For this review, use the dimensioned drawing (mm, ordinates from the lowest corner) and the shaded views. A direction names the side the tool comes from. Coordinates: 2 decimals unless noted, no trailing zeros. Write each loop counter-clockwise with the first axis right and the second up, starting at its lowest first coordinate (ties: lowest second). Pieces come first, ordered by that corner, then holes.
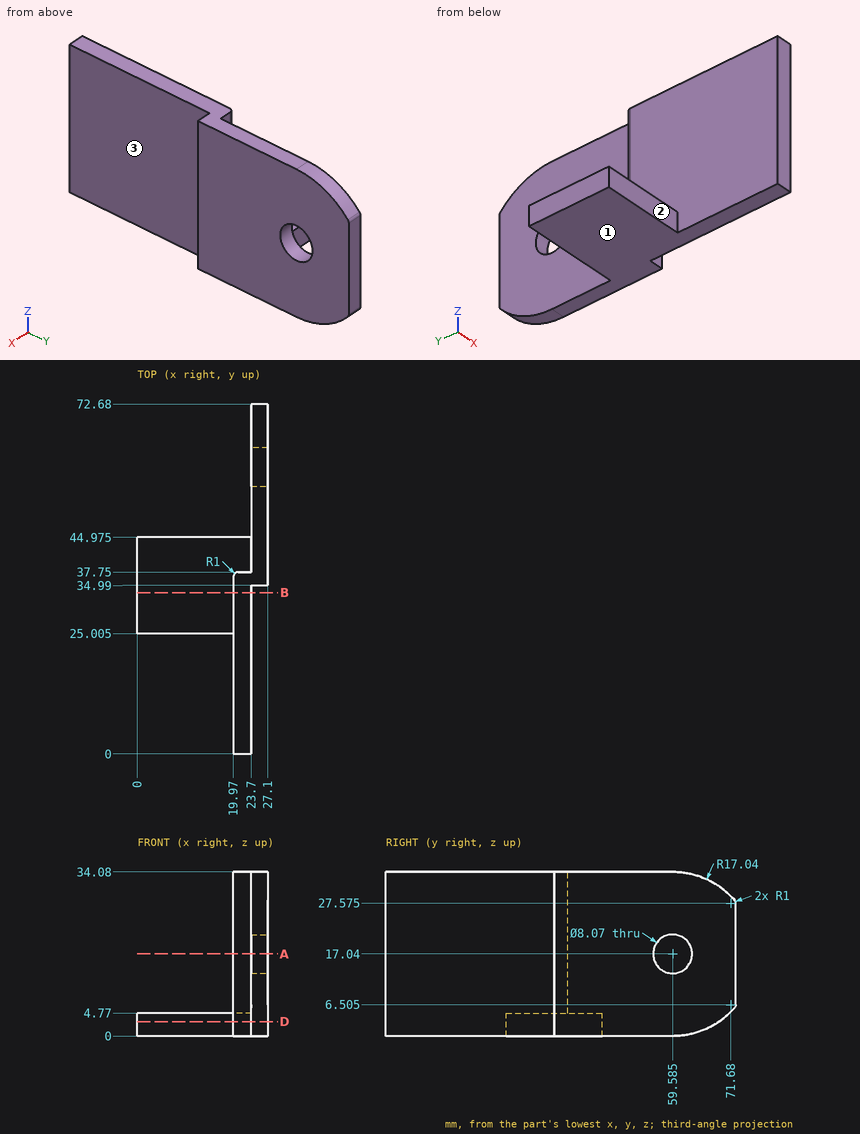
Item 1: Take a section at B-B, the plane y = 33.5. Write out the cut boundary in (x, z), plus the area to 3 significant figures.
Solved:
outline: (0, 0) - (23.7, 0) - (23.7, 34.08) - (19.97, 34.08) - (19.97, 4.77) - (0, 4.77) - close
area: 222 mm2
Item 2: Take a section at A-A, the plane z = 17.04. Write out the cut boundary in (x, y).
Solved:
outline: (19.97, 0) - (23.7, 0) - (23.7, 34.99) - (27.1, 34.99) - (27.1, 55.55) - (23.7, 55.55) - (23.7, 37.75) - (20.97, 37.75) arc R1 ccw to (19.97, 36.75) - close; (23.7, 63.62) - (27.1, 63.62) - (27.1, 72.68) - (23.7, 72.68) - close
Item 3: Take a section at D-D, the plane z = 3. Write out the cut boundary in (x, y) (1 decimal).
Solved:
outline: (0, 25) - (20, 25) - (20, 0) - (23.7, 0) - (23.7, 35) - (27.1, 35) - (27.1, 69.2) - (23.7, 69.2) - (23.7, 45) - (0, 45) - close
Item 4: To check wall thickness, follow line 1 along X through (y, z) = (6.5, 3.5); line 2 along X through (y, z) = (41, 20.5); line 3 along Y through (x, z) = (22.5, 13). State the ranges of each line that lie inside material, in increasing order.
Solved:
line 1: x = 19.97 to 23.7
line 2: x = 23.7 to 27.1
line 3: y = 0 to 37.75
Item 5: Machinability: for the marked faces 1, 2 and 3, which of the approach directions +Z, -Z, +X, -X, +Y, -Y give a long, thin tool a straight path to every point of the face, cutting with its end or side? Answer none if there is none.
Solved:
face 1: -Z, +X, -X, +Y, -Y
face 2: +Z, -Z, -X, -Y
face 3: +Z, -Z, +X, -Y
Item 6: For pin 1 (10 mm diameter, centred on y = 16.5, z = 17.5, fed in from +X); pin 2 (10 mm diameter, centred on y = 32.5, z = 10.5, fed in from -X); pin 3 (2.5 mm diameter, centred on x = 6.5, z = 2.5, fed in from -Y) (3 decimals), all flat-tipped, find the tip position at first contact; note any pin that passes through.
Solved:
pin 1: stops at x = 23.7
pin 2: stops at x = 19.97
pin 3: stops at y = 25.005
